Can you work these out from the model? Positions are in its coordinate system, mm. Face numbers are marked on the shaded views. A direction names the side the tool comes from. Give positions to 0.01 mm unless a question says otherwise; leave off trailing zeros. Order: outer loops, then holes, each group sorted by start corner. A loop starts at its lowest first (then second) coordinate and runs counter-clockwise, first axis right, second up. Notation, with made-up numbers: (66, 19.25) - (115, 19.25) arc R25 ccw to (115, 41.25) - close; hole circle Ø9 at (11.5, -20.75). An arc over 180 degrees is marked (long way). Answer as a JSON object with one key per item and string values.
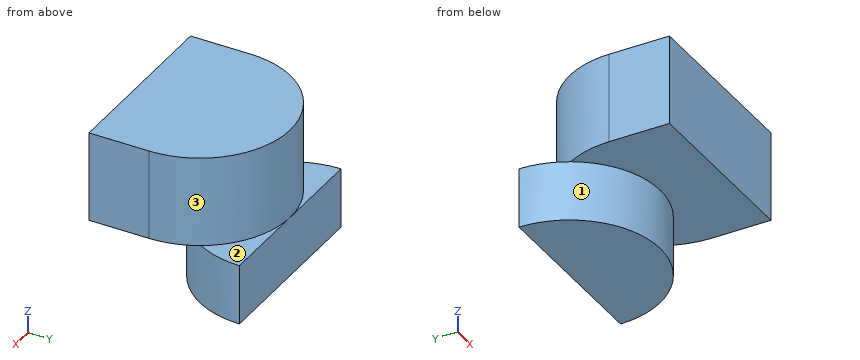
```python
from build123d import *

# Parameters (mm, degrees)
BOSS_EXTRUDE2_DEPTH = 15
BOSS_EXTRUDE3_DEPTH = 10


with BuildPart() as part:
    # Sketch1 → Boss-Extrude2 (new body)
    with BuildSketch(Plane.XY):
        with BuildLine():
            Line((-30, 10), (-30, 0))
            Line((-30, 0), (0, 0))
            Line((0, 0), (0, 10))
            ThreePointArc((0, 10), (-15, 25), (-30, 10))
        make_face()
    extrude(amount=BOSS_EXTRUDE2_DEPTH)

    # Sketch2 → Boss-Extrude3 (add)
    with BuildSketch(Plane(origin=(0, 0, 0), x_dir=(-1, 0, 0), z_dir=(0, 0, -1))):
        with BuildLine():
            Line((0, 25), (30, 25))
            ThreePointArc((30, 25), (15, 10), (0, 25))
        make_face()
    extrude(amount=BOSS_EXTRUDE3_DEPTH)


solid = part.part
```
Q1. If we section it at D-D, the plane x = -22: Please give me the cut outline in (y, z), then the cut area to 3 significant figures.
Recorded:
{"outline": "(0, 0) - (11.73, 0) - (11.73, -10) - (25, -10) - (25, 0) - (23.27, 0) - (23.27, 15) - (0, 15) - close", "area": "482 mm^2"}
Q2. If we section it at C-C, the plane y = 6: Please give me the cut outline in (x, z), then the cut area to 3 significant figures.
Recorded:
{"outline": "(-30, 0) - (0, 0) - (0, 15) - (-30, 15) - close", "area": "450 mm^2"}
Q3. I'm going to push flat-ended pins straight in: pin 1 Ø1.5 at (x, z) = (-14.5, -5.5) entering from -Y; pin 2 Ø5 at (y, z) = (10.5, -5) entering from +X; pin 3 Ø1.5 at (x, z) = (-23, -1.5) entering from -Y. Where does each tip first touch, or does it pass through?
Recorded:
{"pin 1": "stops at y = 10", "pin 2": "stops at x = -6", "pin 3": "stops at y = 11.87"}
Q4. If we section it at A-A, the plane x = -3: Please give me the cut outline in (y, z), then the cut area to 3 significant figures.
Recorded:
{"outline": "(0, 0) - (16, 0) - (16, -10) - (25, -10) - (25, 0) - (19, 0) - (19, 15) - (0, 15) - close", "area": "375 mm^2"}
Q5. Which directions (+Z, -Z, +X, -X, +Y, -Y) give clear straight access to the entire face, cutting with the end or side of a thin tool? Please do the marked faces 1, 2 and 3.
Recorded:
{"face 1": "-Z, -Y", "face 2": "+Z, +X, +Y", "face 3": "+Z, +Y"}
Q6. If we section it at B-B, the plane z = -1: Please give me the cut outline in (x, y).
Recorded:
{"outline": "(-30, 25) arc R15 ccw to (0, 25) - close"}
Q7. I need wall thicknesses on L1, parallel to Y at x = -15, z = -8; L2, parallel to Z at x = -8.75, y = 5.75; L3, parallel to Z at x = -27.25, y = 22. Which ranges of each line are inside material? Lowest first, please.
Recorded:
{"L1": "y = 10 to 25", "L2": "z = 0 to 15", "L3": "z = -10 to 0"}
